```python
from build123d import *

# Parameters (mm, degrees)
SKETCH_1_R          = 5
EXTRUDE_1_DEPTH     = 104
SKETCH_2_W          = 3.498862739
SKETCH_2_H          = 1
CHAMFER_1_SIZE      = 0.5
SKETCH_4_W          = 44.49282487
SKETCH_4_H          = 52.981234512
CUT_EXTRUDE_2_DEPTH = 5


with BuildPart() as part:
    # 草图1 → 拉伸1 (new body)
    with BuildSketch(Plane.XY):
        with Locations(Location((0, 0, 0), (0, 0, 180))):
            Circle(SKETCH_1_R)
    extrude(amount=EXTRUDE_1_DEPTH)

    # 草图2 → 切除-旋转1 (revolve, cut)
    with BuildSketch(Plane(origin=(0, 0, 0), x_dir=(1, 0, 0), z_dir=(0, 1, 0)), mode=Mode.PRIVATE) as cut_revolve_1_sk:
        with Locations((6.39943137, -41)):
            Rectangle(SKETCH_2_W, SKETCH_2_H)
    revolve(cut_revolve_1_sk.sketch.rotate(Axis((0, 0, 104), (0, 0, -1)), 180), axis=Axis((0, 0, 104), (0, 0, -1)), mode=Mode.SUBTRACT)

    # 倒角1
    chamfer_1_edges = [part.edges().sort_by_distance(p)[0] for p in [
        (5, 0, 0),
        (5, 0, 104),
    ]]
    chamfer(chamfer_1_edges, length=CHAMFER_1_SIZE)

    # 草图4 → 拉伸2 (cut, symmetric)
    with BuildSketch(Plane(origin=(0, 0, 0), x_dir=(1, 0, 0), z_dir=(0, 1, 0))):
        with Locations((6.93564623, -90.490617256)):
            Rectangle(SKETCH_4_W, SKETCH_4_H)
    extrude(amount=CUT_EXTRUDE_2_DEPTH, both=True, mode=Mode.SUBTRACT)


solid = part.part
```
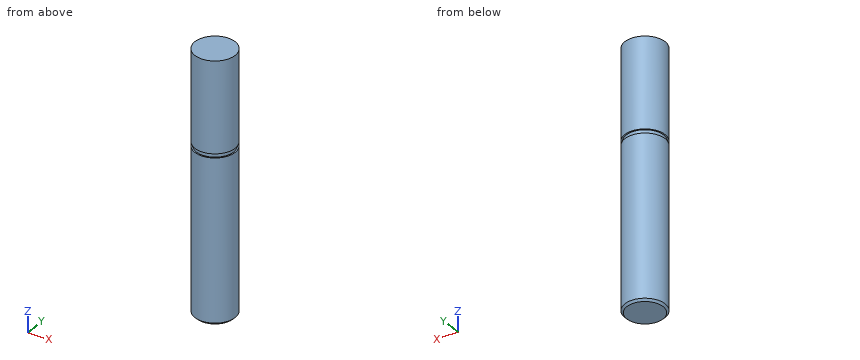
The listing builds one solid part. Answer for the finished solid, in the listing's coordinates (mm). Give positions to 0.01 mm unless a question says otherwise; leave off trailing zeros. Loops run counter-clockwise (first coordinate to the right, second up) from the corner with the lowest first, then second, coordinate; pieces in that order, holes last. Notation, with made-up numbers: M 56.25,59 L 107.25,59 A22 ccw 107.25,91 Z; hole C -5.5,77 d5. An arc over 180 degrees is marked long. One line per item, written item: value.
Q1. Find the intervals of material crossed by line 1 (X direction, y = -0.25, z = 46.5); line 2 (X direction, y = -0.75, z = 27); line 3 (Y direction, x = 3, z = 17.5), in increasing order. Write a range as from..to.
Working result:
line 1: x = -4.99..4.99
line 2: x = -4.94..4.94
line 3: y = -4..4
Q2. A cutting plane is placed at A-A on z = 56. Determine the outline of the cut face in (x, y).
Working result:
outline: C 0,0 d10
Q3. Flat-ended cylindrical pins translate along their axes: P1, Ø3, axis at x = -0.5, y = -1.5, coming from the -Z side; P2, Ø1.5, axis at y = -1, z = 28, coming from the -X side; P3, Ø1, axis at y = -1, z = 15, coming from the +X side; P4, Ø1.5, axis at y = 2, z = 21, coming from the +X side. Find the tip coordinate at first contact, or state that the pin passes through.
Working result:
P1: stops at z = 0
P2: stops at x = -4.99
P3: stops at x = 4.97
P4: stops at x = 4.84
